The model under review builds one solid part; all positions refer to its coordinate system, in mm. A direction names the side the tool comes from. Coordinates: 2 decimals unless noted, no trailing zeros. Loops run counter-clockwise (first coordinate to the right, second up) from the corner with the lowest first, then second, coordinate; pieces in that order, holes last. Notation, with made-up numbers: (-10, 40.25) - (45, 40.25) arc R23 ccw to (45, 54.25) - close; hole circle Ø9 at (-32, 45). An arc over 180 degrees is marked (long way). One line per item, written item: value. Start each with the question number.
1. Insertion check: P1, Ø4, axis at y = 23, z = -15, coming from the -X side; P2, Ø10, axis at y = 28, z = 51, coming from the +X side; P3, Ø17.5, axis at x = -16, z = -15, coming from the +Y side. Each pin has a flat end and moves straight along its axis. Give the tip position at first contact, or say it passes through.
2. For faces 1 (the face through (-2, 35, -60)), 2 (the face through (-5, 23, -1)), list the 3-axis set-ups (+Z, -Z, +X, -X, +Y, -Y) from which the entire face can be reached by the end or side of a thin tool; tool diameter is ignored.
3. We need section D-D, the plane y = 13.5. Give the boundary of the cut face in (x, z), then the cut area to 3 significant figures.
4. We need section C-C, the plane z = 53.5. Give the boundary of the cut face in (x, y).
5. We need section B-B, the plane z = -38. Give the boundary of the cut face in (x, y), then the cut area to 3 significant figures.
6. We need section A-A, the plane y = 20. Give the boundary of the cut face in (x, z), then the cut area to 3 significant figures.
7. Mouldability with a two-part tool opening along Y and no side actions: class faces 3 (the face through (-2, 40, 4)), 4 (the face through (-3, 17, -42)), 5 (the face through (-35, 3, -60)) as +Y half, -Y half, draft (parallel to the pull), parting line (faces both ways), or undercut.
8. To check wall thickness, follow line 1 (Y direction, x = -2.7, z = -38); line 2 (Y direction, x = -7, z = 35); line 3 (X direction, y = 36.5, z = 42). State the ranges of each line that lie inside material, in increasing order.
from build123d import *

# Parameters (mm, degrees)
EXTRUDE_THIN1_DEPTH      = 65
EXTRUDE_THIN1_DEPTH_BACK = 65
CHAMFER1_SIZE            = 10
SKETCH3_R                = 5
CUT_EXTRUDE1_DEPTH       = 10


with BuildPart() as part:
    # Sketch2 → Extrude-Thin1 (new, two sides: drawn at the far end of the back side and taken through both)
    with BuildSketch(Plane.XY.offset(-EXTRUDE_THIN1_DEPTH_BACK)):
        Polygon((-40, 0), (0, 0), (0, 40), (-5, 40), (-5, 5), (-40, 5), align=None)
    extrude(amount=EXTRUDE_THIN1_DEPTH + EXTRUDE_THIN1_DEPTH_BACK)

    # Chamfer1
    chamfer1_edges = [part.edges().sort_by_distance(p)[0] for p in [
        (-40, 2.5, -65),
        (-2.5, 40, -65),
    ]]
    chamfer(chamfer1_edges, length=CHAMFER1_SIZE)

    # Sketch3 → Cut-Extrude1 (cut)
    with BuildSketch(Plane.ZY.offset(5)):
        with Locations((-38, 20)):
            Circle(SKETCH3_R)
    extrude(amount=-CUT_EXTRUDE1_DEPTH, mode=Mode.SUBTRACT)


solid = part.part
Findings below:
1. P1: x = -5
1. P2: x = 0
1. P3: y = 5
2. face 1: -Z, +X, -X, +Y
2. face 2: +Z, -Z, -X, +Y
3. outline: (-5, -65) - (0, -65) - (0, 65) - (-5, 65) - close
3. area: 650 mm2
4. outline: (-40, 0) - (0, 0) - (0, 40) - (-5, 40) - (-5, 5) - (-40, 5) - close
5. outline: (-40, 0) - (0, 0) - (0, 15) - (-5, 15) - (-5, 5) - (-40, 5) - close; (-5, 25) - (0, 25) - (0, 40) - (-5, 40) - close
5. area: 325 mm2
6. outline: (-5, -65) - (0, -65) - (0, -43) - (-5, -43) - close; (-5, -33) - (0, -33) - (0, 65) - (-5, 65) - close
6. area: 600 mm2
7. face 3: +Y half
7. face 4: undercut
7. face 5: draft
8. line 1: 0 to 15, 25 to 40
8. line 2: 0 to 5
8. line 3: -5 to 0
